Geometry: final body of the model. Coordinates: model frame, mm. A direction names the side the tool comes from. Give positions to 0.01 mm unless a question says otherwise; leave off trailing zeros. Write each loop counter-clockwise with the first axis right and the second up, starting at its lowest first coordinate (ties: lowest second). Pieces come first, ordered by that corner, then holes. Notation, with made-up numbers: M -24.75,31 L 12.25,31 A23 cw 12.25,65 Z; hole C 46,-13.5 d5. An arc over 180 degrees is marked long. Use a Markdown table: item, result. Add a question column.
(1) Pin query (flat end, axial travel): pin 1 Ø10 at (x, y) = (63.5, -0.5) entering from +Z; pin 2 Ø20 at (y, z) = (-42.5, 74.5) entering from +X. Return the tip coordinate at first contact, or that it passes through.
(2) Cut plane A-A (y = -24). Output: boundary loops of the cut face in (x, z), plus the area to 3 significant figures.
(3) Material intervals for L1, parallel to Z at x = 15, y = -38.5; L2, parallel to Y at x = 22, z = 58.5; L3, parallel to X at y = -18, z = 81, sorted ascending.
(4) Cut plane C-C (x = 79.5). Output: boundary loops of the cut face in (y, z), plus the area to 3 significant figures.
(5) Reachability of faces 1 (the flat face through (15, -3, 0)), 2 (the flat face through (-24.327, -34, 75)) from +Z, -Z, +X, -X, +Y, -Y: full face, straight path, thin tool, end or side. Return the list, or none.
(6) Cut plane B-B (x = 3). Output: boundary loops of the cut face in (y, z), plus the area to 3 significant figures.
```python
from build123d import *

# Parameters (mm, degrees)
F0_W     = 150
F0_H     = 100
F1_DEPTH = 50
F2_W     = 35
F2_H     = 100
F3_DEPTH = 50
F4_W     = 85
F4_H     = 60
F5_DEPTH = 50
F7_DEPTH = 60


with BuildPart() as f1:
    # F0 (on Top) → F1 (new body)
    with BuildSketch(Plane.XY):
        with Locations((15.672885, -3.26121)):
            Rectangle(F0_W, F0_H)
    extrude(amount=F1_DEPTH)

    # F2 (on face) → F3 (join)
    with BuildSketch(Plane.XY.offset(50)):
        with Locations((-41.827115, -3.26121)):
            Rectangle(F2_W, F2_H)
    extrude(amount=F3_DEPTH)

    # F4 (on face) → F5 (join)
    with BuildSketch(Plane.XY.offset(50)):
        with Locations((18.172885, 16.73879)):
            Rectangle(F4_W, F4_H)
    extrude(amount=F5_DEPTH)

    # F6 (on face) → F7 (cut)
    with BuildSketch(Plane.XZ.offset(13.26121)):
        Polygon((60.672885, 100), (-24.327115, 100), (60.672885, 50), align=None)
    extrude(amount=-F7_DEPTH, mode=Mode.SUBTRACT)


solid = f1.part
```
Answer list:
| question | item | result |
|---|---|---|
| 1 | pin 1 | z = 51.28 |
| 1 | pin 2 | x = -24.33 |
| 2 | outline | M -59.33,0 L 90.67,0 L 90.67,50 L -24.33,50 L -24.33,100 L -59.33,100 Z |
| 2 | area | 9,250 mm² |
| 3 | L1 | 0 to 50 |
| 3 | L2 | -13.26 to 46.74 |
| 3 | L3 | -59.33 to -24.33 |
| 4 | outline | M -53.26,0 L 46.74,0 L 46.74,50 L -53.26,50 Z |
| 4 | area | 5,000 mm² |
| 5 | face 1 | -Z, +X, -X, +Y, -Y |
| 5 | face 2 | +Z, +X, -Y |
| 6 | outline | M -53.26,0 L 46.74,0 L 46.74,83.93 L -13.26,83.93 L -13.26,50 L -53.26,50 Z |
| 6 | area | 7,040 mm² |
